```python
from build123d import *

# Parameters (mm, degrees)
BOSS_EXTRUDE1_DEPTH = 1
SKETCH4_R           = 1.5
CUT_EXTRUDE5_DEPTH  = 1
SKETCH5_R           = 5
BOSS_EXTRUDE2_DEPTH = 40


with BuildPart() as part:
    # Sketch1 → Boss-Extrude1 (new body)
    with BuildSketch(Plane.XY):
        Polygon((-20, 35), (-20, -40), (0, -40), (0, 0), (15, 15), (55, 15), (55, 35), align=None)
    extrude(amount=BOSS_EXTRUDE1_DEPTH)

    # Sketch4 → Cut-Extrude5 (cut)
    with BuildSketch(Plane.XY.offset(1)):
        with Locations((-10, 25.000149563)):
            Circle(SKETCH4_R)
    extrude(amount=-CUT_EXTRUDE5_DEPTH, mode=Mode.SUBTRACT)

    # Sketch5 → Boss-Extrude2 (add)
    with BuildSketch(Plane.XY.offset(1)):
        with Locations(Location((43.007008147, 25, 0), (0, 0, 180))):
            Circle(SKETCH5_R)
    extrude(amount=BOSS_EXTRUDE2_DEPTH)


solid = part.part
```
Work out the finished part from the listing and answer in its coordinate system (mm). Give positions to 0.01 mm unless a question says otherwise; leave off trailing zeros. Order: outer loops, then holes, each group sorted by start corner. A loop starts at its lowest first (then second) coordinate and runs counter-clockwise, first axis right, second up. Notation, with made-up numbers: (-5.75, -3.75) - (36.25, -3.75) arc R6 ccw to (36.25, 5.25) - close; hole circle Ø7 at (-19.75, 76). An arc over 180 degrees is marked (long way). One line per item, written item: value. Start each with the question number.
1. Section C-C, the plane z = 3.5 is taken. Write down the section's boundary in (x, y).
2. For a pull along X with two mould halves and no side action, classify faces 1 (the face through (0, 15, 1)), 2 (the face through (-10.195, 26.487, 0.507)), 3 (the face through (7.4, 7.4, 0.5)), 4 (the face through (40.7, 29.436, 20.72)) as released by +X, released by -X, zero draft, split by the parting line, or undercut.
3. Section B-B, the plane y = -30.5 is taken. Write down the section's boundary in (x, z).
4. Section A-A, the plane x = -10 is taken. Write down the section's boundary in (y, z), then the cut area to 3 significant figures.
5. Consider line 1 (Y direction, x = -10, z = 0.5); line 2 (Z direction, x = 22, y = 23); line 3 (X direction, y = 29, z = 32.5). Determine where each line is inside the solid, lowest interval first.
6. Section D-D, the plane x = 41 is taken. Write down the section's boundary in (y, z).
7. Each of these flat-tipped pins is pushed along its axis until it touches: pin 1 Ø1.1 at (x, z) = (43, 0.5) entering from -Y; pin 2 Ø0.8 at (y, z) = (-29.5, 0.5) entering from +X; pin 3 Ø6 at (x, y) = (-2.5, 22) entering from +Z. Where does it stop, or does it pass through?
Filled sheet:
1. outline: circle Ø10 at (43.01, 25)
2. face 1: zero draft
2. face 2: undercut
2. face 3: released by +X
2. face 4: split by the parting line
3. outline: (-20, 0) - (0, 0) - (0, 1) - (-20, 1) - close
4. outline: (-40, 0) - (23.5, 0) - (23.5, 1) - (-40, 1) - close; (26.5, 0) - (35, 0) - (35, 1) - (26.5, 1) - close
4. area: 72.0 mm²
5. line 1: -40 to 23.5, 26.5 to 35
5. line 2: 0 to 1
5. line 3: 40.01 to 46.01
6. outline: (15, 0) - (35, 0) - (35, 1) - (29.58, 1) - (29.58, 41) - (20.42, 41) - (20.42, 1) - (15, 1) - close
7. pin 1: y = 15
7. pin 2: x = 0
7. pin 3: z = 1
